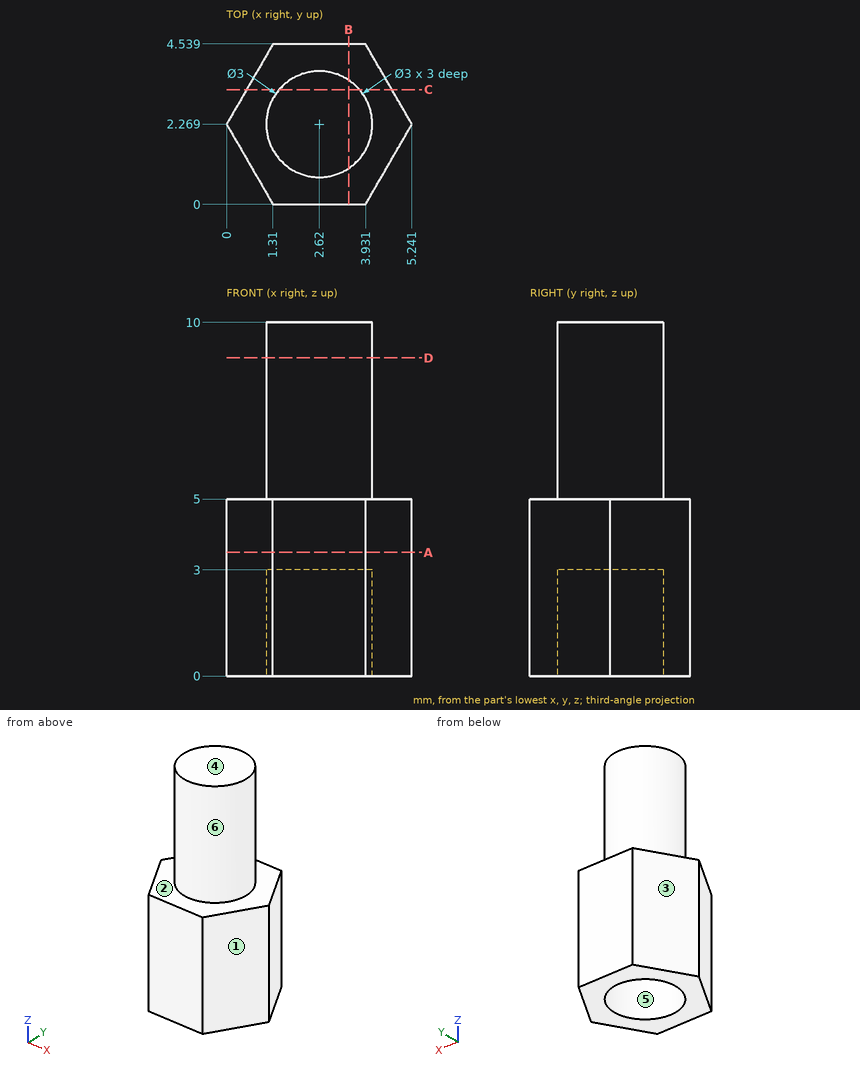
Part print with two shaded views. Sizes in mm from the minimum x, y, z corner. A direction names the side the tool comes from. Round coordinates to 2 decimals unless told otherwise and drop trailing zeros. Order: outer loops, then holes, each group sorted by start corner. A loop starts at its lowest first (then second) coordinate and runs counter-clockwise, first axis right, second up. Notation, with made-up numbers: M -2.75,37 L 3.25,37 A26 cw 3.25,73 Z; hole C 13,27 d6. An arc over 180 degrees is marked long. Use CSV: the item, a comma, the result in double quotes. Start each with the question number.
(1) Cut at C-C on y = 3.25. List the corners of the cut face in (x, z) (1 decimal).
(2) Cut at D-D on z = 9. List the corners of the cut face in (x, y).
(3) Tool access for the marked faces 1 and 2: list every direction of +Z, -Z, +X, -X, +Y, -Y with a clear straight run to the whole face (end or side of a thin tool).
(4) Flat gauge pins, fed straight in: P1, Ø1.5, axis at y = 2.5, z = 6, coming from the +X side; P2, Ø2, axis at x = 3, z = 8.5, coming from the -Y side. Where does each tip first touch, or does it go through?
(5) Cut at A-A on z = 3.5. List the corners of the cut face in (x, y).
(6) Drill centre lines: probe 1 along Z at (x, y) = (4.1, 0.75); probe 2 along Y at (x, z) = (2.7, 6); probe 3 along Z at (x, y) = (3.2, 1.25). Where is each one in solid material? Low to high.
(7) Mould opens along X. For the marked faces 3, 4, 5 and 6 say: +X half, -X half, draft (parallel to the pull), parting line (faces both ways), or undercut.
(8) Cut at B-B on x = 3.45. List the corners of the cut face in (y, z).
Findings:
1,outline,"M 0.6,0 L 1.5,0 L 1.5,3 L 3.8,3 L 3.8,0 L 4.7,0 L 4.7,5 L 3.8,5 L 3.8,10 L 1.5,10 L 1.5,5 L 0.6,5 Z"
2,outline,"C 2.62,2.27 d3"
3,face 1,"+Z, -Z, +X, -Y"
3,face 2,"+Z"
4,P1,"stops at x = 4.12"
4,P2,"stops at y = 0.77"
5,outline,"M 0,2.27 L 1.31,0 L 3.93,0 L 5.24,2.27 L 3.93,4.54 L 1.31,4.54 Z"
6,probe 1,"z = 0 to 5"
6,probe 2,"y = 0.77 to 3.77"
6,probe 3,"z = 3 to 10"
7,face 3,"-X half"
7,face 4,"draft"
7,face 5,"undercut"
7,face 6,"parting line"
8,outline,"M 0,0 L 1.02,0 L 1.02,3 L 3.52,3 L 3.52,0 L 4.54,0 L 4.54,5 L 3.52,5 L 3.52,10 L 1.02,10 L 1.02,5 L 0,5 Z"
